Check sheet for the modelled part. Datum: model origin and axes. Units: mm. Round coordinates to 2 decimals unless told otherwise and drop trailing zeros. Write each loop counter-clockwise with the first axis right and the second up, starting at its lowest first coordinate (ties: lowest second). Pieces come first, ordered by that corner, then holes. Notation, with made-up numbers: (70.25, 17.5) - (122.25, 17.5) arc R24 cw to (122.25, 33.5) - close; hole circle Ø11 at (9, 14). An arc over 180 degrees is marked (long way). Answer as a JSON object with one key per item and string values. Group by question number.
Item 1: Sectioned sample at A-A on y = 1.55. Record the boundary of the cut face in (x, z), plus the area to 3 significant figures.
Item 2: Sectioned sample at B-B on z = 7.5. Record the boundary of the cut face in (x, y).
Item 3: Release check for a two-part mould opening along X. For faces 1 (the flat face through (0, 1, -20)), 2 (the flat face through (13, 1.2, 0)), 3 (the flat face through (-35, 1, 0)) record: pulls with the +X half, pulls with the -X half, needs draft (parallel to the pull), parting line crosses it, or undercut.
Item 4: Thickness scan on line 1 (X direction, y = 1.95, z = -8.5). Record the ranges inside material, lowest first.
Autodesk Inventor part; units mm, degrees
ref_plane "YZ Plane" through (0, 0, 0) normal (1, 0, 0) x (0, 1, 0)
ref_plane "XZ Plane" through (0, 0, 0) normal (0, 1, 0) x (-1, 0, 0)
ref_plane "XY Plane" through (0, 0, 0) normal (0, 0, 1) x (1, 0, 0)
sketch "Эскиз1" plane through (0, 0, 0) normal (0, 1, 0) x (-1, 0, 0)
  line L0 (-35, -20) -> (35, -20)
  line L1 (35, -20) -> (35, 20)
  line L2 (35, 20) -> (-35, 20)
  line L3 (-35, 20) -> (-35, -20)
  line L4 (-35, -20) -> (35, 20) construction
  line L5 (35, -20) -> (-35, 20) construction
  point P0 (0, 0)
  dimension "d0" = 70
  dimension "d1" = 40
extrude "Выдавливание1" add sketch "Эскиз1" along normal blind 2.2
sketch "Эскиз2" plane through (0, 2.2, 0) normal (0, 1, 0) x (1, 0, 0)
  line L0 (-35, -20) -> (35, -20)
  line L1 (35, 20) -> (-35, 20)
  line L2 (12.0013, -20) -> (14.8088, -20)
  line L3 (14.8088, -20) -> (14.8088, 20)
  line L4 (14.8088, 20) -> (12.0013, 20)
  line L5 (12.0013, 20) -> (12.0013, -20)
  point P0 (0, 0)
extrude "Выдавливание2" cut sketch "Эскиз2" against normal blind 1
properties part number "test"
Completed:
{
 "1": {"outline": "(-35, -20) - (12, -20) - (12, 20) - (-35, 20) - close; (14.81, -20) - (35, -20) - (35, 20) - (14.81, 20) - close", "area": "2,690 mm²"},
 "2": {"outline": "(-35, 0) - (35, 0) - (35, 2.2) - (14.81, 2.2) - (14.81, 1.2) - (12, 1.2) - (12, 2.2) - (-35, 2.2) - close"},
 "3": {"face 1": "needs draft", "face 2": "undercut", "face 3": "pulls with the -X half"},
 "4": {"line 1": "-35 to 12, 14.81 to 35"}
}
